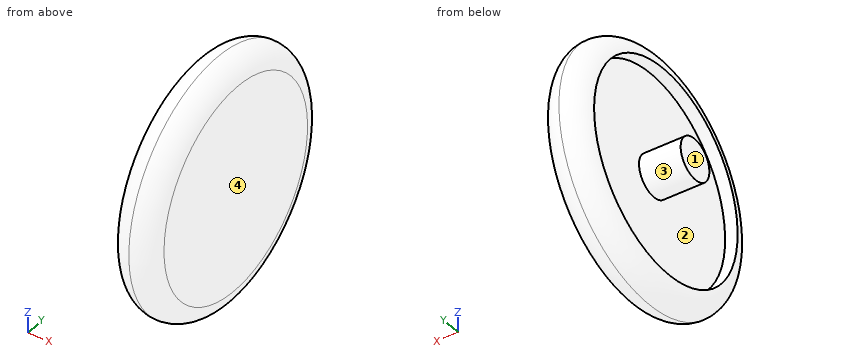
```python
from build123d import *

# Parameters (mm, degrees)
FILLET1_R = 5


with BuildPart() as part:
    # Sketch1 → Revolve2 (revolve)
    with BuildSketch(Plane.XY, mode=Mode.PRIVATE) as revolve2_sk:
        Polygon((0, 0), (0, 5), (10, 5), (10, 25), (7, 25), (7, 30), (17, 30), (17, 0), align=None)
    revolve(revolve2_sk.sketch.rotate(Axis((0, 0, 0), (1, 0, 0)), 90), axis=Axis((0, 0, 0), (1, 0, 0)))

    # Fillet1
    fillet1_edges = [part.edges().sort_by_distance(p)[0] for p in [
        (7, 0, -30),
        (17, 0, -30),
    ]]
    fillet(fillet1_edges, radius=FILLET1_R - 0.0001)  # a hair under: the kernel refuses the full size


solid = part.part
```
Can you work these out from the model? Positions are in its coordinate system, mm. Face numbers are marked on the shaded views. A direction names the side the tool comes from. Round coordinates to 2 decimals unless told otherwise and drop trailing zeros. Loops run counter-clockwise (first coordinate to the right, second up) from the corner with the lowest first, then second, coordinate; pieces in that order, holes last. Notation, with made-up numbers: M 65,-20 L 91,-20 A22 cw 91,3 Z; hole C -29,14.5 d6. An arc over 180 degrees is marked long. Answer as a JSON object with one key per item and string values. Group by question number.
Q1. Please list where these lines run through material, in increasing order: L1, parallel to X at y = 2.5, z = 7; L2, parallel to Z at x = 8.75, y = 3; L3, parallel to Y at x = 8.35, z = 0.
Q2. Imagine slicing it at D-D, the plane x = 1.5. Please give me the cut outline in (y, z).
Q3. Imagine slicing it at C-C, the plane x = 9.25. Please give me the cut outline in (y, z), then the cut area to 3 significant figures.
Q4. We'd pull the mould along Y, two halves only. Please class the marked faces 1 and 2: +Y half, -Y half, draft (parallel to the pull), parting line (faces both ways), or undercut.
Q5. Will these pins go through, and if not, where does the flat tip stop? pin 1 (6 mm diameter, centred on x = 2.5, y = -20.5, fed in from -Z); pin 2 (1 mm diameter, centred on x = 14.5, z = 11.5, fed in from +Y); pin 3 (15 mm diameter, centred on y = 5.5, z = 8, fed in from -X); pin 4 (3 mm diameter, centred on x = 4, z = -0.5, fed in from +Y).
Q6. On a 3-axis mill with a long thin cutter (end or side, diameter ignored), from which of +Z, -Z, +X, -X, +Y, -Y can I reach the whole of each face in a straight line? I mean the marked faces 3 and 4. Say none if no direction works.
Findings:
{
 "1": {"L1": "x = 10 to 17", "L2": "z = -28.64 to -24.82, -4 to 4, 24.82 to 28.64", "L3": "y = -28.42 to -25, -5 to 5, 25 to 28.42"},
 "2": {"outline": "C 0,0 d10"},
 "3": {"outline": "C 0,0 d58.35; C 0,0 d10; hole C 0,0 d50", "area": "789 mm2"},
 "4": {"face 1": "draft", "face 2": "undercut"},
 "5": {"pin 1": "passes through", "pin 2": "stops at y = 27.33", "pin 3": "stops at x = 0", "pin 4": "stops at y = 5"},
 "6": {"face 3": "-X", "face 4": "+Z, -Z, +X, +Y, -Y"}
}
